Geometry check sheet. Reference: the model listing, model coordinates, mm. Face numbers are marked on the shaded views. A direction names the side the tool comes from. Give positions to 0.01 mm unless a question says otherwise; leave off trailing zeros. Loops run counter-clockwise (first coordinate to the right, second up) from the corner with the lowest first, then second, coordinate; pieces in that order, holes last. Notation, with made-up numbers: (2.25, 35.5) -> (9.25, 35.5) arc R21 cw to (9.25, 62.5) -> close; hole circle Ø3 at (23.5, 37.5). An arc over 180 degrees is marked (long way). Answer as a JSON object with one key per item and string values.
from build123d import *

# Parameters (mm, degrees)
F0_W      = 28.5392315894
F0_H      = 48.2956362042
F1_DEPTH  = 25.4
F1_FACE_W = 28.5392315894
F1_FACE_H = 48.2956362042
F2_ANGLE  = 90
F3_DEPTH  = 25.4
F4_W      = 26.9696157947
F4_H      = 26.9696157947
F5_DEPTH  = 50.14334
F8_W      = 6.35
F8_H      = 25.4
F9_DEPTH  = 25.4
F10_R     = 2.5796875
F11_DEPTH = 50.8
F13_DEPTH = 12.7
F15_DEPTH = 6.35
F16_DEPTH = 50.8


with BuildPart() as f1:
    # F0 (on Front) → F1 (new body)
    with BuildSketch(Plane.XZ):
        with Locations((-3.175, -0.3527777778)):
            Rectangle(F0_W, F0_H)
        Polygon((-12.7, -19.4027777778), (-12.7, 18.6972222222), (6.35, 18.6972222222), (6.35, 2.8222222222), (-1.27, 2.8222222222), (-1.27, -3.5277777778), (6.35, -3.5277777778), (6.35, -19.4027777778), align=None, mode=Mode.SUBTRACT)
    extrude(amount=F1_DEPTH)

    # F1_face (on face) → F2 (revolve)
    with BuildSketch(Plane(origin=(-2.7804632911, -25.4, -0.3527777778), x_dir=(1, 0, 0), z_dir=(0, -1, 0))):
        with Locations((-0.3945367089, 0)):
            Rectangle(F1_FACE_W, F1_FACE_H)
        Polygon((9.1304632911, -19.05), (-9.9195367089, -19.05), (-9.9195367089, 19.05), (9.1304632911, 19.05), (9.1304632911, 3.175), (1.5104632911, 3.175), (1.5104632911, -3.175), (9.1304632911, -3.175), align=None, mode=Mode.SUBTRACT)
    revolve(axis=Axis((11.0946157947, -25.4, -0.3527777778), (0, 0, 1)), revolution_arc=F2_ANGLE)

    # F3 (add): a face of the model
    f3_faces = [f1.faces().sort_by_distance(p)[0] for p in [
        (11.0946157947, -22.3630131274, -0.3527777778),
    ]]
    extrude(f3_faces, amount=F3_DEPTH)

    # F4 (on face) → F5 (cut, symmetric)
    with BuildSketch(Plane(origin=(0, 0, -24.5005958799), x_dir=(1, 0, 0), z_dir=(0, 0, -1))):
        with Locations((23.0098078974, 13.4848078974)):
            Rectangle(F4_W, F4_H)
    extrude(amount=F5_DEPTH, both=True, mode=Mode.SUBTRACT)

    # F8 (on face) + F6 (on face) → F9 (join)
    with BuildSketch(Plane(origin=(0, 0, -24.5005958799), x_dir=(1, 0, 0), z_dir=(0, 0, -1))):
        with Locations((-14.2696157947, 12.7)):
            Rectangle(F8_W, F8_H)
        with Locations((6.35, 12.7)):
            Rectangle(F8_W, F8_H)
    with BuildSketch(Plane(origin=(0, 0, -24.5005958799), x_dir=(1, 0, 0), z_dir=(0, 0, -1))):
        with BuildLine():
            Line((9.525, 0), (9.525, 26.9696157947))
            Line((9.525, 26.9696157947), (9.5198247534, 33.3196136858))
            Line((9.5198247534, 33.3196136858), (36.4946157947, 33.3415981335))
            Line((36.4946157947, 33.3415981335), (36.4946157947, 47.5892315894))
            Line((36.4946157947, 47.5892315894), (9.5198157947, 47.5892315894))
            Line((9.5198157947, 47.5892315894), (9.5198157947, 53.8957495896))
            ThreePointArc((9.5198157947, 53.8957495896), (-9.6349683982, 45.0156080432), (-17.4446157947, 25.4))
            Line((-17.4446157947, 25.4), (-17.4446157947, 0))
            Line((-17.4446157947, 0), (9.525, 0))
        make_face()
        with BuildLine():
            Line((9.5198157947, 47.5892315894), (36.4946157947, 47.5892315894))
            Line((36.4946157947, 47.5892315894), (36.4946157947, 53.9392315894))
            Line((36.4946157947, 53.9392315894), (11.0946157947, 53.9392315894))
            ThreePointArc((11.0946157947, 53.9392315894), (10.3069157052, 53.9283590184), (9.5198157947, 53.8957495896))
            Line((9.5198157947, 53.8957495896), (9.5198157947, 47.5892315894))
        make_face()
        Polygon((9.5198247534, 33.3196136858), (9.525, 26.9696157947), (36.4946157947, 26.9915960246), (36.4946157947, 33.3415981335), align=None)
    extrude(amount=F9_DEPTH)

    # F10 (on face) → F11 (cut)
    with BuildSketch(Plane(origin=(-17.4446157947, 0, 0), x_dir=(0, -1, 0), z_dir=(-1, 0, 0))):
        with Locations((12.7, -35.9203596757)):
            Circle(F10_R)
    extrude(amount=-F11_DEPTH, mode=Mode.SUBTRACT)

    # F12 (on face) → F13 (join)
    with BuildSketch(Plane(origin=(0, 0, 0), x_dir=(-1, 0, 0), z_dir=(0, 1, 0))):
        Polygon((-9.525, 23.7950403243), (-9.525, -0.3527777778), (-9.525, -49.9005958799), (17.4446157947, -49.9005958799), (17.4446157947, 23.7950403243), align=None)
        Polygon((1.27, -3.5277777778), (1.27, -0.3527777778), (1.27, 2.8222222222), (-6.35, 2.8222222222), (-6.35, 18.6972222222), (12.7, 18.6972222222), (12.7, -19.4027777778), (-6.35, -19.4027777778), (-6.35, -3.5277777778), align=None, mode=Mode.SUBTRACT)
    extrude(amount=F13_DEPTH)

    # F15 (add): a face of the model
    f15_faces = [f1.faces().sort_by_distance(p)[0] for p in [
        (4.9144212495, -24.754718946, -49.9005958799),
    ]]
    extrude(f15_faces, amount=F15_DEPTH)

    # F14 (on face) → F16 (cut)
    with BuildSketch(Plane(origin=(-17.4446157947, 0, 0), x_dir=(0, -1, 0), z_dir=(-1, 0, 0))):
        with BuildLine():
            Line((-7.9248, -35.6191955507), (10.1379524268, -35.6191955507))
            ThreePointArc((10.1379524268, -35.6191955507), (12.7, -33.3406721757), (15.2620475732, -35.6191955507))
            Line((15.2620475732, -35.6191955507), (20.6248, -35.6191955507))
            ThreePointArc((20.6248, -35.6191955507), (6.35, -21.3443955507), (-7.9248, -35.6191955507))
        make_face()
        with BuildLine():
            Line((12.7, -48.4038510032), (12.7, -38.5000471757))
            ThreePointArc((12.7, -38.5000471757), (10.772346384, -37.634693113), (10.1379524268, -35.6191955507))
            Line((10.1379524268, -35.6191955507), (-7.9248, -35.6191955507))
            ThreePointArc((-7.9248, -35.6191955507), (-1.1708023189, -47.7521031791), (12.7, -48.4038510032))
        make_face()
        with BuildLine():
            ThreePointArc((15.2796875, -35.9203596757), (14.5241145246, -37.7444742003), (12.7, -38.5000471757))
            Line((12.7, -38.5000471757), (12.7, -48.4038510032))
            ThreePointArc((12.7, -48.4038510032), (18.4829076284, -43.1399978696), (20.6248, -35.6191955507))
            Line((20.6248, -35.6191955507), (15.2620475732, -35.6191955507))
            ThreePointArc((15.2620475732, -35.6191955507), (15.2752737424, -35.7695195308), (15.2796875, -35.9203596757))
        make_face()
    extrude(amount=-F16_DEPTH, mode=Mode.SUBTRACT)


solid = f1.part
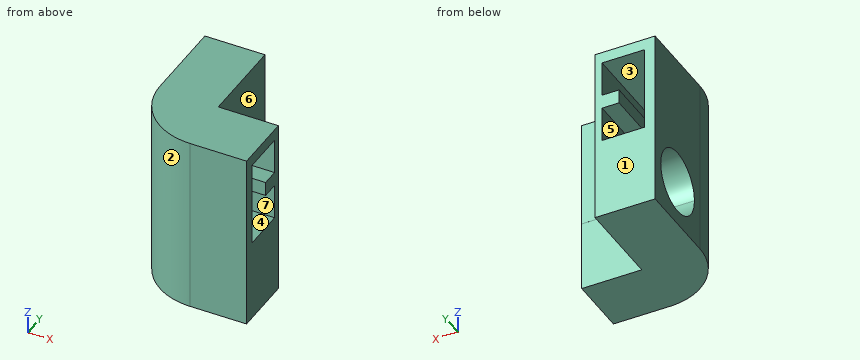
1) Tool access check on the marked faces 4, 5, 6 and 7. Record the directions out of +Z, -Z, +X, -X, +Y, -Y that give a thin tool (end or side, any length) a straight path to the whole face; none if there is none.
Geometry check:
{"face 4": "none", "face 5": "+Y", "face 6": "+Z, -Z, +X, +Y", "face 7": "+X"}
2) Section check B-B on z = 6.5. Record the cut outline in (x, y) (3 decimals), plus the area to 3 significant figures.
Geometry check:
{"outline": "(-17.445, -25.4) arc R28.539 ccw to (11.095, -53.939) -> (36.495, -53.939) -> (36.495, -49.195) -> (11.095, -49.195) arc R23.795 cw to (-12.7, -25.4) -> (-12.7, 12.7) -> (-17.445, 12.7) -> close; (6.35, -25.4) arc R4.745 ccw to (11.095, -30.145) -> (36.495, -30.145) -> (36.495, -26.97) -> (9.525, -26.97) -> (9.525, 12.7) -> (6.35, 12.7) -> close", "area": "713 mm2"}
3) Depth check by flat-ended pin: P1, Ø19, axis at x = 23.5, y = -4.5, coming from the -Z side; P2, Ø13.5, axis at x = 19, z = -10.5, coming from the +Y side; P3, Ø4, axis at x = 1, z = 3.5, coming from the -Y side; P4, Ø12, axis at y = -9.5, z = -26.5, coming from the +X side (3 decimals). Enter the tip coordinate at first touch or a pass-through.
Geometry check:
{"P1": "passes through", "P2": "stops at y = -26.97", "P3": "stops at y = -52.77", "P4": "stops at x = 9.525"}
4) Section check A-A on y = -6.35. Record the cut outline in (x, z) (3 decimals), plus the area to 3 significant figures.
Geometry check:
{"outline": "(-17.445, -56.251) -> (9.525, -56.251) -> (9.525, -49.894) -> (-17.445, -49.894) -> close; (-17.445, -21.344) -> (9.525, -21.344) -> (9.525, 23.795) -> (-17.445, 23.795) -> close; hole (-12.7, -19.403) -> (6.35, -19.403) -> (6.35, -3.528) -> (-1.27, -3.528) -> (-1.27, 2.822) -> (6.35, 2.822) -> (6.35, 18.697) -> (-12.7, 18.697) -> close", "area": "711 mm2"}
5) Draft check along X on the marked faces 1, 2 and 3. Enter one of: pulls with the +X half, pulls with the -X half, needs draft (parallel to the pull), parting line crosses it, or undercut.
Geometry check:
{"face 1": "needs draft", "face 2": "pulls with the -X half", "face 3": "undercut"}
6) Section check D-D on x = -3. Record the cut outline in (y, z).
Geometry check:
{"outline": "(-50.22, -56.25) -> (12.7, -56.25) -> (12.7, -19.4) -> (-44.57, -19.4) -> (-44.57, 18.7) -> (12.7, 18.7) -> (12.7, 23.8) -> (-50.22, 23.8) -> close; hole circle Ø28.55 at (-6.35, -35.62)"}
7) Material ranges on line 1 along X through (y, z) = (-10.5, 6) (3 decimals); line 2 along Z through (x, y) = (9.5, -46); line 3 along X through (y, z) = (-26, -2.5) (3 decimals), recorded low to high. Write a range as from..to.
Geometry check:
{"line 1": "x = -17.445..-12.7, 6.35..9.525", "line 2": "z = -56.25..-19.4, 18.7..23.8", "line 3": "x = -17.438..-12.692, -1.255..9.525"}
8) Section check C-C on y = -23.5. Record the cut outline in (x, z) (3 decimals), plus the area to 3 significant figures.
Geometry check:
{"outline": "(-17.445, -56.251) -> (9.525, -56.251) -> (9.525, 23.795) -> (-17.445, 23.795) -> close; hole (-12.7, -19.403) -> (6.35, -19.403) -> (6.35, -3.528) -> (-1.27, -3.528) -> (-1.27, 2.822) -> (6.35, 2.822) -> (6.35, 18.697) -> (-12.7, 18.697) -> close", "area": "1,480 mm2"}
